from build123d import *

# Parameters (mm, degrees)
SKETCH3_W                          = 100.33
SKETCH3_H                          = 63.5
BOSS_EXTRUDE3_DEPTH                = 39.37
SKETCH5_OUTSIDE_W                  = 93.994
SKETCH5_OUTSIDE_H                  = 109.234
SKETCH5_OUTSIDE_R                  = 31.75
CUT_EXTRUDE1_DEPTH                 = 44.45
SKETCH6_R                          = 18
CUT_EXTRUDE2_DEPTH                 = 132.431194927
BOSS_EXTRUDE4_DEPTH                = 19.05
CUT_EXTRUDE3_START                 = -0.254
SKETCH12_W                         = 63.5
SKETCH12_H                         = 34.8
CUT_EXTRUDE3_DEPTH                 = 0.254
F_5_16_18_TAPPED_HOLE1_D           = 6.5278
F_5_16_18_TAPPED_HOLE1_DEPTH       = 20.1168
F_5_16_18_TAPPED_HOLE1_CSINK_D     = 9.2075
F_5_16_18_TAPPED_HOLE1_CSINK_ANGLE = 90
F_5_16_18_TAPPED_HOLE1_TIP         = 1.961148974
F_1_4_20_TAPPED_HOLE2_AT_2_COUNT   = 2
F_1_4_20_TAPPED_HOLE2_AT_2_PITCH   = 43.510583459
F_1_4_20_TAPPED_HOLE2_AT_3_COUNT   = 2
F_1_4_20_TAPPED_HOLE2_AT_3_PITCH   = 17.771582008
F_1_4_20_TAPPED_HOLE2_AT_4_COUNT   = 2
F_1_4_20_TAPPED_HOLE2_AT_4_PITCH   = 18.200222467
F_1_4_20_TAPPED_HOLE2_AT_5_COUNT   = 2
F_1_4_20_TAPPED_HOLE2_AT_5_PITCH   = 43.333034767
F_1_4_20_TAPPED_HOLE2_AT_6_COUNT   = 2
F_1_4_20_TAPPED_HOLE2_AT_6_PITCH   = 46.999427507
F_1_4_20_TAPPED_HOLE3_AT_2_COUNT   = 2
F_1_4_20_TAPPED_HOLE3_AT_2_PITCH   = 33.655


with BuildPart() as part:
    # Sketch3 → Boss-Extrude3 (new, symmetric)
    with BuildSketch(Plane(origin=(0, 0, 0), x_dir=(1, 0, 0), z_dir=(0, 1, 0))):
        with Locations((50.165, 0)):
            Rectangle(SKETCH3_W, SKETCH3_H)
    extrude(amount=BOSS_EXTRUDE3_DEPTH, both=True)

    # Sketch5 outside → Cut-Extrude1 (cut)
    with BuildSketch(Plane.ZY):
        Rectangle(SKETCH5_OUTSIDE_W, SKETCH5_OUTSIDE_H)
        Circle(SKETCH5_OUTSIDE_R, mode=Mode.SUBTRACT)
    extrude(amount=-CUT_EXTRUDE1_DEPTH, mode=Mode.SUBTRACT)

    # Sketch6 → Cut-Extrude2 (cut, through all)
    with BuildSketch(Plane(origin=(0, 39.37, 0), x_dir=(1, 0, 0), z_dir=(0, 1, 0))):
        with Locations(Location((76.2, 0, 0), (0, 0, 270))):
            Circle(SKETCH6_R)
    extrude(amount=-CUT_EXTRUDE2_DEPTH, mode=Mode.SUBTRACT)

    # Sketch9 → Boss-Extrude4 (add)
    with BuildSketch(Plane.ZY):
        with BuildLine():
            Line((-15.24, 11.05), (15.24, 11.05))
            ThreePointArc((15.24, 11.05), (26.29, 0), (15.24, -11.05))
            Line((15.24, -11.05), (-15.24, -11.05))
            ThreePointArc((-15.24, -11.05), (-26.29, 0), (-15.24, 11.05))
        make_face()
    extrude(amount=BOSS_EXTRUDE4_DEPTH)

    # Sketch12 → Cut-Extrude3 (cut)
    with BuildSketch(Plane.ZY.offset(CUT_EXTRUDE3_START)):
        Rectangle(SKETCH12_W, SKETCH12_H)
        with BuildLine():
            Line((-15.24, -11.05), (15.24, -11.05))
            ThreePointArc((15.24, -11.05), (26.29, 0), (15.24, 11.05))
            Line((15.24, 11.05), (-15.24, 11.05))
            ThreePointArc((-15.24, 11.05), (-26.29, 0), (-15.24, -11.05))
        make_face(mode=Mode.SUBTRACT)
    extrude(amount=CUT_EXTRUDE3_DEPTH, mode=Mode.SUBTRACT)

    # 5/16-18 Tapped Hole1
    with Locations(Plane.ZY.offset(19.05)):
        with Locations((-15.24, 0), (15.24, 0)):
            CounterSinkHole(F_5_16_18_TAPPED_HOLE1_D / 2, F_5_16_18_TAPPED_HOLE1_CSINK_D / 2, depth=F_5_16_18_TAPPED_HOLE1_DEPTH, counter_sink_angle=F_5_16_18_TAPPED_HOLE1_CSINK_ANGLE)
            with Locations((0, 0, -(F_5_16_18_TAPPED_HOLE1_DEPTH + F_5_16_18_TAPPED_HOLE1_TIP / 2))):  # 118° drill point
                Cone(0, F_5_16_18_TAPPED_HOLE1_D / 2, F_5_16_18_TAPPED_HOLE1_TIP, mode=Mode.SUBTRACT)

    # Sketch7 → 1/4-20 Tapped Hole2 (revolve, cut)
    with BuildSketch(Plane(origin=(76.431975719, 39.37, -23.49885502), x_dir=(0, 0, 1), z_dir=(1, 0, 0))):
        Polygon((0, 0), (0, 18.043816902), (2.5527, 16.51), (2.5527, 1.2573), (3.81, 0), align=None)
    f_1_4_20_tapped_hole2 = revolve(axis=Axis((76.431975719, 45.72, -23.49885502), (0, -1, 0)), mode=Mode.SUBTRACT)

    # 1/4-20 Tapped Hole2 at 2: 1/4-20 Tapped Hole2 ×2
    with Locations(*[Vector(-0.38723877589339034, 0, 0.9219794631360227) * (i * F_1_4_20_TAPPED_HOLE2_AT_2_PITCH) for i in range(1, F_1_4_20_TAPPED_HOLE2_AT_2_COUNT)]):
        add(f_1_4_20_tapped_hole2, mode=Mode.SUBTRACT)

    # 1/4-20 Tapped Hole2 at 3: 1/4-20 Tapped Hole2 ×2
    with Locations(*[Vector(0.9219794631360225, 0, 0.3872387758933909) * (i * F_1_4_20_TAPPED_HOLE2_AT_3_PITCH) for i in range(1, F_1_4_20_TAPPED_HOLE2_AT_3_COUNT)]):
        add(f_1_4_20_tapped_hole2, mode=Mode.SUBTRACT)

    # 1/4-20 Tapped Hole2 at 4: 1/4-20 Tapped Hole2 ×2
    with Locations(*[Vector(-0.9257570948708089, 0, 0.37811876612561857) * (i * F_1_4_20_TAPPED_HOLE2_AT_4_PITCH) for i in range(1, F_1_4_20_TAPPED_HOLE2_AT_4_COUNT)]):
        add(f_1_4_20_tapped_hole2, mode=Mode.SUBTRACT)

    # 1/4-20 Tapped Hole2 at 5: 1/4-20 Tapped Hole2 ×2
    with Locations(*[Vector(0.37811876612561857, 0, 0.9257570948708089) * (i * F_1_4_20_TAPPED_HOLE2_AT_5_PITCH) for i in range(1, F_1_4_20_TAPPED_HOLE2_AT_5_COUNT)]):
        add(f_1_4_20_tapped_hole2, mode=Mode.SUBTRACT)

    # 1/4-20 Tapped Hole2 at 6: 1/4-20 Tapped Hole2 ×2
    with Locations(*[Vector(-0.004935713719611744, 0, 0.9999878192908542) * (i * F_1_4_20_TAPPED_HOLE2_AT_6_PITCH) for i in range(1, F_1_4_20_TAPPED_HOLE2_AT_6_COUNT)]):
        add(f_1_4_20_tapped_hole2, mode=Mode.SUBTRACT)

    # Mirror1: 1/4-20 Tapped Hole2 across plane
    add(f_1_4_20_tapped_hole2.mirror(Plane.ZX), mode=Mode.SUBTRACT)

    # Mirror1 copy 1 sketch → Mirror1 copy 1 (revolve, cut)
    with BuildSketch(Plane(origin=(59.582990642, -39.37, 16.617009358), x_dir=(0, 0, 1), z_dir=(1, 0, 0))):
        Polygon((0, 0), (0, -18.043816902), (2.5527, -16.51), (2.5527, -1.2573), (3.81, 0), align=None)
    revolve(axis=Axis((59.582990642, -45.72, 16.617009358), (0, -1, 0)), mode=Mode.SUBTRACT)

    # Mirror1 copy 2 sketch → Mirror1 copy 2 (revolve, cut)
    with BuildSketch(Plane(origin=(92.817009358, -39.37, -16.617009358), x_dir=(0, 0, 1), z_dir=(1, 0, 0))):
        Polygon((0, 0), (0, -18.043816902), (2.5527, -16.51), (2.5527, -1.2573), (3.81, 0), align=None)
    revolve(axis=Axis((92.817009358, -45.72, -16.617009358), (0, -1, 0)), mode=Mode.SUBTRACT)

    # Mirror1 copy 3 sketch → Mirror1 copy 3 (revolve, cut)
    with BuildSketch(Plane(origin=(59.582990642, -39.37, -16.617009358), x_dir=(0, 0, 1), z_dir=(1, 0, 0))):
        Polygon((0, 0), (0, -18.043816902), (2.5527, -16.51), (2.5527, -1.2573), (3.81, 0), align=None)
    revolve(axis=Axis((59.582990642, -45.72, -16.617009358), (0, -1, 0)), mode=Mode.SUBTRACT)

    # Mirror1 copy 4 sketch → Mirror1 copy 4 (revolve, cut)
    with BuildSketch(Plane(origin=(92.817009358, -39.37, 16.617009358), x_dir=(0, 0, 1), z_dir=(1, 0, 0))):
        Polygon((0, 0), (0, -18.043816902), (2.5527, -16.51), (2.5527, -1.2573), (3.81, 0), align=None)
    revolve(axis=Axis((92.817009358, -45.72, 16.617009358), (0, -1, 0)), mode=Mode.SUBTRACT)

    # Mirror1 copy 5 sketch → Mirror1 copy 5 (revolve, cut)
    with BuildSketch(Plane(origin=(76.2, -39.37, 23.5), x_dir=(0, 0, 1), z_dir=(1, 0, 0))):
        Polygon((0, 0), (0, -18.043816902), (2.5527, -16.51), (2.5527, -1.2573), (3.81, 0), align=None)
    revolve(axis=Axis((76.2, -45.72, 23.5), (0, -1, 0)), mode=Mode.SUBTRACT)

    # Sketch13 → 1/4-20 Tapped Hole3 (revolve, cut)
    with BuildSketch(Plane(origin=(53.975, 29.845, 31.75), x_dir=(0, -1, 0), z_dir=(1, 0, 0))):
        Polygon((0, 0), (0, 18.043816902), (2.5527, 16.51), (2.5527, 1.2573), (3.81, 0), align=None)
    f_1_4_20_tapped_hole3 = revolve(axis=Axis((53.975, 29.845, 38.1), (0, 0, -1)), mode=Mode.SUBTRACT)

    # 1/4-20 Tapped Hole3 at 2: 1/4-20 Tapped Hole3 ×2
    with Locations(*[(i * F_1_4_20_TAPPED_HOLE3_AT_2_PITCH, 0, 0) for i in range(1, F_1_4_20_TAPPED_HOLE3_AT_2_COUNT)]):
        add(f_1_4_20_tapped_hole3, mode=Mode.SUBTRACT)

    # Mirror2: 1/4-20 Tapped Hole3 across plane
    add(f_1_4_20_tapped_hole3.mirror(Plane.XY), mode=Mode.SUBTRACT)

    # Mirror2 copy 1 sketch → Mirror2 copy 1 (revolve, cut)
    with BuildSketch(Plane(origin=(87.63, 29.845, -31.75), x_dir=(0, -1, 0), z_dir=(1, 0, 0))):
        Polygon((0, 0), (0, -18.043816902), (2.5527, -16.51), (2.5527, -1.2573), (3.81, 0), align=None)
    revolve(axis=Axis((87.63, 29.845, -38.1), (0, 0, -1)), mode=Mode.SUBTRACT)


solid = part.part
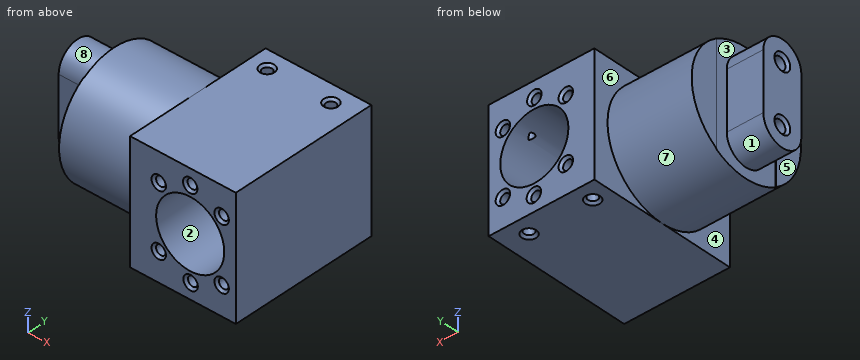
The listing builds one solid part. Answer for the finished solid, in the listing's coordinates (mm). Face numbers are marked on the shaded views. A direction names the side the tool comes from. Give positions to 0.01 mm unless a question says otherwise; leave off trailing zeros. Write each loop counter-clockwise with the first axis right and the second up, starting at its lowest first coordinate (ties: lowest second). Pieces come first, ordered by that corner, then holes. Notation, with made-up numbers: (48, 40) - (60, 40) arc R33 ccw to (60, 74) - close; hole circle Ø10 at (74.25, 22). An arc over 180 degrees is marked (long way). One line per question, with ' | ' between items. Start each with the question number.
1. Straight lines are drawn through the part: line 1 (Z direction, x = -9.75, y = 0); line 2 (Y direction, x = -7, z = 15); line 3 (X direction, y = 11.5, z = 0.5). For each, find the intervals that lie inside material, in ascending order.
2. Given P1, Ø7, axis at y = 26.5, z = -3, coming from the -X side; P2, Ø6.5, axis at x = 76.2, z = 23.5, coming from the -Y side; P3, Ø6.5, axis at x = 53.975, y = 29.845, coming from the -Z side, each flat-ended and moving along its own axis, determine where each tip first touches the part or whether it passes through.
3. Section B-B, the plane y = -8 is taken. Determine the outline of the cut face in (x, z), then the cut area to 3 significant figures.
4. For the marked faces 4, 5, 6, 7 and 8, determine the directions among +Z, -Z, +X, -X, +Y, -Y from which every point of the face is accessible in a straight line to the end or side of a thin tool.
5. Section C-C, the plane x = 19.5 is taken. Determine the outline of the cut face in (y, z), then the cut area to 3 significant figures.
6. Section A-A, the plane z = 0 is taken. Determine the outline of the cut face in (x, y).
7. Determine the mould class of the marked faces 1, 2 and 3 for opening direction X: +X half, -X half, draft (parallel to the pull), parting line (faces both ways), or undercut.
Result:
1) line 1: z = -26.29 to -18.5, -11.98 to 11.98, 18.5 to 26.29 | line 2: y = -11.05 to -3.26, 3.26 to 11.05 | line 3: x = 0.25 to 58.21, 94.19 to 100.33
2) P1: stops at x = 0 | P2: stops at y = -38.81 | P3: stops at z = -31.19
3) outline: (-19.05, -22.86) - (0.25, -22.86) - (0.25, -30.73) - (44.45, -30.73) - (44.45, -31.75) - (100.33, -31.75) - (100.33, 31.75) - (44.45, 31.75) - (44.45, 30.73) - (0.25, 30.73) - (0.25, 22.86) - (-19.05, 22.86) - close; hole circle Ø36 at (76.2, 0) | area: 6,130 mm2
4) face 4: -X, -Y | face 5: +Z, -Z, -X, -Y | face 6: -X, +Y | face 7: -X | face 8: +Z, -X
5) outline: circle Ø63.5 at (0, 0) | area: 3,170 mm2
6) outline: (-19.05, -11.05) - (0.25, -11.05) - (0.25, -17.4) - (0, -17.4) - (0, -31.75) - (44.45, -31.75) - (44.45, -39.37) - (58.2, -39.37) - (58.2, 39.37) - (44.45, 39.37) - (44.45, 31.75) - (0, 31.75) - (0, 17.4) - (0.25, 17.4) - (0.25, 11.05) - (-19.05, 11.05) - close; (94.2, -39.37) - (100.33, -39.37) - (100.33, 39.37) - (94.2, 39.37) - close
7) face 1: draft | face 2: undercut | face 3: -X half
